from build123d import *

# Parameters (mm, degrees)
SKETCH1_W           = 46
SKETCH1_H           = 10
BOSS_EXTRUDE1_DEPTH = 4
SKETCH4_W           = 27
SKETCH4_H           = 8
BOSS_EXTRUDE2_DEPTH = 16
SKETCH5_R           = 1.600993429
SKETCH5_R_2         = 1.598160281
CUT_EXTRUDE2_DEPTH  = 16
SKETCH6_R           = 1.494820838
SKETCH6_R_2         = 1.5
CUT_EXTRUDE3_DEPTH  = 16
FILLET1_R           = 5


with BuildPart() as part:
    # Sketch1 → Boss-Extrude1 (new body)
    with BuildSketch(Plane.XY):
        with Locations((23, 5)):
            Rectangle(SKETCH1_W, SKETCH1_H)
    extrude(amount=BOSS_EXTRUDE1_DEPTH)

    # Sketch4 → Boss-Extrude2 (add)
    with BuildSketch(Plane.XY.offset(4)):
        with Locations((13.5, 6)):
            Rectangle(SKETCH4_W, SKETCH4_H)
    extrude(amount=BOSS_EXTRUDE2_DEPTH)

    # Sketch5 → Cut-Extrude2 (cut)
    with BuildSketch(Plane.XZ.offset(-2)):
        with Locations((22.999560123, 14.235930167)):
            Circle(SKETCH5_R)
        with Locations((5.001441553, 14.237615424)):
            Circle(SKETCH5_R_2)
    extrude(amount=-CUT_EXTRUDE2_DEPTH, mode=Mode.SUBTRACT)

    # Sketch6 → Cut-Extrude3 (cut)
    with BuildSketch(Plane(origin=(0, 0, 0), x_dir=(-1, 0, 0), z_dir=(0, 0, -1))):
        with Locations((-42, 5)):
            Circle(SKETCH6_R)
        with Locations((-29.333333333, 5)):
            Circle(SKETCH6_R_2)
        with Locations((-35.666666667, 5)):
            Circle(SKETCH6_R_2)
    extrude(amount=-CUT_EXTRUDE3_DEPTH, mode=Mode.SUBTRACT)

    # Fillet1
    fillet1_edges = [part.edges().sort_by_distance(p)[0] for p in [
        (0, 6, 20),
        (27, 6, 20),
    ]]
    fillet(fillet1_edges, radius=FILLET1_R)


solid = part.part
Design review of the part built by this model. Coordinates are the model's own, in mm. A direction names the side the tool comes from. Coordinates: 2 decimals unless noted, no trailing zeros. Order: outer loops, then holes, each group sorted by start corner. A loop starts at its lowest first (then second) coordinate and runs counter-clockwise, first axis right, second up.
Item 1: Take a section at B-B, the plane y = 5.75. Write out the cut boundary in (x, z).
Item 2: For pin 1 Ø1 at (x, y) = (31.5, 7) entering from +Z; pin 2 Ø1.8 at (x, y) = (35.67, 5) entering from +Z; pin 3 Ø5 at (x, z) = (5, 14.24) entering from -Y, all flat-tipped, find the tip position at first contact; note any pin that passes through.
Item 3: Take a section at C-C, the plane z = 2. Write out the cut boundary in (x, y), then the cut area to 3 significant figures.
Item 4: Take a section at D-D, the plane x = 6. Write out the cut boundary in (y, z).
Item 5: The part is to be moulded in two halves that separate along Y. For faces 4 (the flat face through (18, 10, 8)), 5 (the cylindrical face through (43.493, 5.066, 1.972)), 6 (the flat face through (23, 0, 2)), say which applies: pulls with the +Y half, pulls with the -Y half, needs draft (parallel to the pull), parting line crosses it, or undercut.
Item 6: For faces 1 (the flat face through (27, 6, 9)), 2 (the flat face through (13, 6, 20)), 3 (the flat face through (13, 2, 12)), list the 3-axis set-ups (+Z, -Z, +X, -X, +Y, -Y) from which the entire face can be reached by the end or side of a thin tool; tool diameter is ignored.
Item 7: For line 1 (Z direction, x = 5, y = 6); line 2 (X direction, y = 6.25, z = 13.5); line 3 (X direction, y = 2.75, z = 14.5), list the stretches that pass through material, from the lowest coordinate up.
Item 8: Take a section at A-A, the plane x = 42. Write out the cut boundary in (y, z).
The answers:
1. outline: (0, 0) - (28.03, 0) - (28.03, 4) - (27, 4) - (27, 15) arc R5 ccw to (22, 20) - (5, 20) arc R5 ccw to (0, 15) - close; (30.63, 0) - (34.37, 0) - (34.37, 4) - (30.63, 4) - close; (36.97, 0) - (40.71, 0) - (40.71, 4) - (36.97, 4) - close; (43.29, 0) - (46, 0) - (46, 4) - (43.29, 4) - close; hole circle Ø3.2 at (5, 14.24); hole circle Ø3.2 at (23, 14.24)
2. pin 1: stops at z = 4
2. pin 2: passes through
2. pin 3: stops at y = 2
3. outline: (0, 0) - (46, 0) - (46, 10) - (0, 10) - close; hole circle Ø3 at (29.33, 5); hole circle Ø3 at (35.67, 5); hole circle Ø2.99 at (42, 5)
3. area: 439 mm2
4. outline: (0, 0) - (10, 0) - (10, 12.99) - (2, 12.99) - (2, 4) - (0, 4) - close; (2, 15.49) - (10, 15.49) - (10, 20) - (2, 20) - close
5. face 4: pulls with the +Y half
5. face 5: undercut
5. face 6: pulls with the -Y half
6. face 1: +Z, +X, +Y, -Y
6. face 2: +Z, +X, -X, +Y, -Y
6. face 3: +Z, +X, -X, -Y
7. line 1: z = 0 to 12.64, 15.84 to 20
7. line 2: x = 0 to 3.58, 6.42 to 21.58, 24.42 to 27
7. line 3: x = 0 to 3.42, 6.58 to 21.42, 24.58 to 27
8. outline: (0, 0) - (3.51, 0) - (3.51, 4) - (0, 4) - close; (6.49, 0) - (10, 0) - (10, 4) - (6.49, 4) - close
